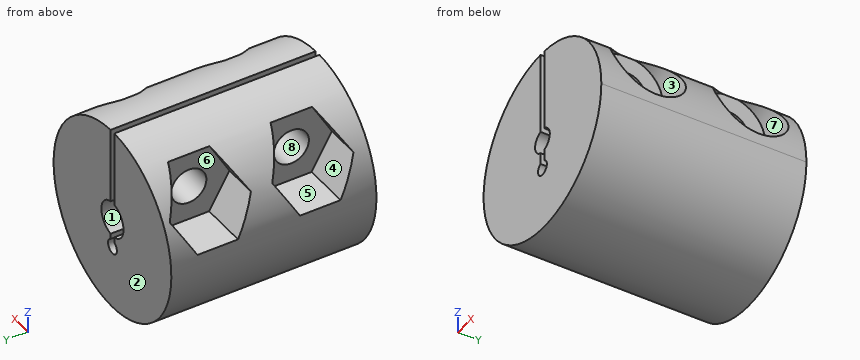
```python
from build123d import *

# Parameters (mm, degrees)
SALIENTE_EXTRUIR1_DEPTH    = 8
SALIENTE_EXTRUIR2_START    = -9.5
SALIENTE_EXTRUIR2_DEPTH    = 9.5
CORTAR_EXTRUIR1_DEPTH      = 15.773286703
CORTAR_EXTRUIR1_DEPTH_BACK = 15.773286703
CROQUIS3_R                 = 1.5
CROQUIS5_R                 = 3
CORTAR_EXTRUIR2_DEPTH      = 4
CORTAR_EXTRUIR4_DEPTH      = 4
CORTAR_EXTRUIR3_DEPTH      = 15.773286703
CORTAR_EXTRUIR3_DEPTH_BACK = 15.773286703
CROQUIS6_OUTSIDE_W         = 23.722
CROQUIS6_OUTSIDE_H         = 23.722
CROQUIS6_OUTSIDE_R         = 8


with BuildPart() as part:
    # Croquis1 → Saliente-Extruir1 (new body)
    with BuildSketch(Plane(origin=(0, 0, 0), x_dir=(1, 0, 0), z_dir=(0, 1, 0))):
        with BuildLine():
            Line((-0.25, -7.996092796), (-0.25, -1.479019946))
            ThreePointArc((-0.25, -1.479019946), (-1.5, 0), (-0.25, 1.479019946))
            Line((-0.25, 1.479019946), (-0.25, 1.954564394))
            ThreePointArc((-0.25, 1.954564394), (0, 3.1), (0.25, 1.954564394))
            Line((0.25, 1.954564394), (0.25, 1.479019946))
            ThreePointArc((0.25, 1.479019946), (1.5, 0), (0.25, -1.479019946))
            Line((0.25, -1.479019946), (0.25, -7.996092796))
            Line((0.25, -7.996092796), (0.25, -8))
            Line((0.25, -8), (8, -8))
            Line((8, -8), (8, 8))
            Line((8, 8), (-8, 8))
            Line((-8, 8), (-8, -8))
            Line((-8, -8), (-0.25, -8))
            Line((-0.25, -8), (-0.25, -7.996092796))
        make_face()
    extrude(amount=SALIENTE_EXTRUIR1_DEPTH)

    # Croquis2 → Saliente-Extruir2 (add)
    with BuildSketch(Plane(origin=(0, 0, 0), x_dir=(1, 0, 0), z_dir=(0, 1, 0)).offset(SALIENTE_EXTRUIR2_START)):
        with BuildLine():
            Line((0.25, -1.479019946), (0.25, -8))
            Line((0.25, -8), (8, -8))
            Line((8, -8), (8, 8))
            Line((8, 8), (-8, 8))
            Line((-8, 8), (-8, -8))
            Line((-8, -8), (-0.25, -8))
            Line((-0.25, -8), (-0.25, -1.479019946))
            Line((-0.25, -1.479019946), (-0.25, -0.968245837))
            ThreePointArc((-0.25, -0.968245837), (-1, 0), (-0.25, 0.968245837))
            Line((-0.25, 0.968245837), (-0.25, 1.479019946))
            Line((-0.25, 1.479019946), (-0.25, 1.954564394))
            ThreePointArc((-0.25, 1.954564394), (0, 3.1), (0.25, 1.954564394))
            Line((0.25, 1.954564394), (0.25, 1.479019946))
            Line((0.25, 1.479019946), (0.25, 0.968245837))
            ThreePointArc((0.25, 0.968245837), (1, 0), (0.25, -0.968245837))
            Line((0.25, -0.968245837), (0.25, -1.479019946))
        make_face()
    extrude(amount=SALIENTE_EXTRUIR2_DEPTH)

    # Croquis3 → Cortar-Extruir1 (cut, two sides: drawn at the far end of the back side and taken through both)
    with BuildSketch(Plane(origin=(0, 0, 0), x_dir=(0, 0, -1), z_dir=(1, 0, 0)).offset(-CORTAR_EXTRUIR1_DEPTH_BACK)):
        with Locations((-4, 4)):
            Circle(CROQUIS3_R)
        with Locations((-4, -4.75)):
            Circle(CROQUIS3_R)
    extrude(amount=CORTAR_EXTRUIR1_DEPTH + CORTAR_EXTRUIR1_DEPTH_BACK, mode=Mode.SUBTRACT)

    # Croquis5 → Cortar-Extruir2 (cut)
    with BuildSketch(Plane(origin=(8, 0, 0), x_dir=(0, 0, -1), z_dir=(1, 0, 0))):
        with Locations((-4, 4)):
            Circle(CROQUIS5_R)
        with Locations((-4, -4.75)):
            Circle(CROQUIS5_R)
    extrude(amount=-CORTAR_EXTRUIR2_DEPTH, mode=Mode.SUBTRACT)

    # Croquis7 → Cortar-Extruir4 (cut)
    with BuildSketch(Plane.ZY.offset(8)):
        Polygon((1, 5.732050808), (1, 2.267949192), (4, 0.535898385), (7, 2.267949192), (7, 5.732050808), (4, 7.464101615), align=None)
        Polygon((1, -3.017949192), (1, -6.482050808), (4, -8.214101615), (7, -6.482050808), (7, -3.017949192), (4, -1.285898385), align=None)
    extrude(amount=-CORTAR_EXTRUIR4_DEPTH, mode=Mode.SUBTRACT)

    # Croquis6 outside → Cortar-Extruir3 (cut, two sides: drawn at the far end of the back side and taken through both)
    with BuildSketch(Plane(origin=(0, 0, 0), x_dir=(1, 0, 0), z_dir=(0, 1, 0)).offset(-CORTAR_EXTRUIR3_DEPTH_BACK)):
        Rectangle(CROQUIS6_OUTSIDE_W, CROQUIS6_OUTSIDE_H)
        Circle(CROQUIS6_OUTSIDE_R, mode=Mode.SUBTRACT)
    extrude(amount=CORTAR_EXTRUIR3_DEPTH + CORTAR_EXTRUIR3_DEPTH_BACK, mode=Mode.SUBTRACT)


solid = part.part
```
Geometry check sheet. Reference: the model listing, model coordinates, mm. Face numbers are marked on the shaded views. A direction names the side the tool comes from. Coordinates: 2 decimals unless noted, no trailing zeros. Loops run counter-clockwise (first coordinate to the right, second up) from the corner with the lowest first, then second, coordinate; pieces in that order, holes last.
Item 1: Go/stop test with flat-tipped pins: pin 1 Ø7.5 at (y, z) = (0, 4) entering from +X; pin 2 Ø1.1 at (y, z) = (-3.5, -1.5) entering from -X; pin 3 Ø1 at (x, y) = (-5.5, 4.5) entering from +Z. Record where each tip stops, or that it passes through.
Item 2: Sectioned sample at B-B, the plane x = -2.75. Record the boundary of the cut face in (y, z).
Item 3: Access from +Z, -Z, +X, -X, +Y, -Y to the whole of each face (thin tool, end or side, straight path). Record for the marked faces 5, 6, 7 and 8.
Item 4: Sectioned sample at A-A, the plane y = -4.75. Record the boundary of the cut face in (x, z).
Item 5: Release check for a two-part mould opening along Y. For the marked faces 1, 2, 3 and 4 record: released by +Y, released by -Y, zero draft, split by the parting line, or undercut.
Item 6: Sectioned sample at D-D, the plane y = 4. Record the boundary of the cut face in (x, z), then the cut area to 3 significant figures.
Item 7: Thickness scan on line 1 (Y direction, x = 2.9, z = 4); line 2 (Y direction, x = 5.7, z = 4); line 3 (X direction, y = -4.25, z = 2.5). Record the ranges inside material, lowest first.
Item 8: Sectioned sample at C-C, the plane z = -2.5. Record the boundary of the cut face in (x, y), then the cut area to 3 significant figures.
Check result:
1. pin 1: stops at x = 8
1. pin 2: stops at x = -7.94
1. pin 3: stops at z = 1
2. outline: (-9.5, -7.51) - (8, -7.51) - (8, 7.51) - (-9.5, 7.51) - close; hole circle Ø3 at (-4.75, 4); hole circle Ø3 at (4, 4)
3. face 5: +Z, -X
3. face 6: -X
3. face 7: +X
3. face 8: +X, -X
4. outline: (-7.94, 1) arc R8 ccw (long way) to (7.94, 1) - (4, 1) - (4, 2.5) - (0.25, 2.5) - (0.25, 0.97) arc R1 cw to (0.25, -0.97) - (0.25, -1.95) arc R0.6 cw (long way) to (-0.25, -1.95) - (-0.25, -0.97) arc R1 cw to (-0.25, 0.97) - (-0.25, 2.5) - (-4, 2.5) - (-4, 1) - close; (-4, 5.5) - (-0.25, 5.5) - (-0.25, 8) arc R8 ccw to (-4, 6.93) - close; (0.25, 5.5) - (4, 5.5) - (4, 6.93) arc R8 ccw to (0.25, 8) - close
5. face 1: zero draft
5. face 2: released by +Y
5. face 3: undercut
5. face 4: undercut
6. outline: (-7.94, 1) arc R8 ccw (long way) to (7.94, 1) - (4, 1) - (4, 2.5) - (0.25, 2.5) - (0.25, 1.48) arc R1.5 cw to (0.25, -1.48) - (0.25, -1.95) arc R0.6 cw (long way) to (-0.25, -1.95) - (-0.25, -1.48) arc R1.5 cw to (-0.25, 1.48) - (-0.25, 2.5) - (-4, 2.5) - (-4, 1) - close; (-4, 5.5) - (-0.25, 5.5) - (-0.25, 8) arc R8 ccw to (-4, 6.93) - close; (0.25, 5.5) - (4, 5.5) - (4, 6.93) arc R8 ccw to (0.25, 8) - close
6. area: 136 mm2
7. line 1: y = -9.5 to -6.25, -3.25 to 2.5, 5.5 to 8
7. line 2: y = -9.5 to -7.75, -1.75 to 1, 7 to 8
7. line 3: x = -4 to -0.25, 0.25 to 4
8. outline: (-7.6, -9.5) - (-0.6, -9.5) - (-0.6, 8) - (-7.6, 8) - close; (0.6, -9.5) - (7.6, -9.5) - (7.6, 8) - (0.6, 8) - close
8. area: 245 mm2
